Geometry check sheet. Reference: the model listing, model coordinates, mm. Face numbers are marked on the shaded views. A direction names the side the tool comes from. Give positions to 0.01 mm unless a question says otherwise; leave off trailing zeros. Order: outer loops, then holes, each group sorted by start corner. A loop starts at its lowest first (then second) coordinate and runs counter-clockwise, first axis right, second up.
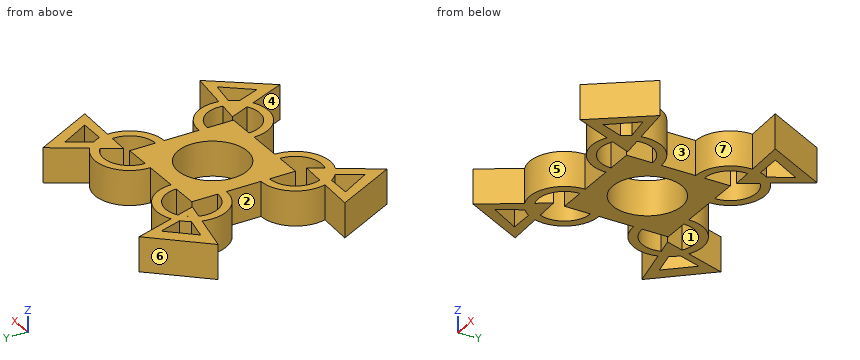
from build123d import *

# Parameters (mm, degrees)
F0_W     = 38.1
F0_H     = 38.1
F0_R     = 12.7
F1_DEPTH = 6.35
F2_R     = 12.7
F2_R_2   = 9.525
F3_DEPTH = 12.7
F5_DEPTH = 12.7


with BuildPart() as f1:
    # F0 (on Top) → F1 (new body, symmetric)
    with BuildSketch(Plane.XY):
        Rectangle(F0_W, F0_H)
        Circle(F0_R, mode=Mode.SUBTRACT)
    extrude(amount=F1_DEPTH, both=True)

    # F2 (on face) → F3 (join)
    with BuildSketch(Plane.XY.offset(6.35)):
        with Locations((-19.05, 19.05)):
            Circle(F2_R)
        with Locations((-19.05, 19.05)):
            Circle(F2_R_2, mode=Mode.SUBTRACT)
        with Locations((19.05, 19.05)):
            Circle(F2_R)
        with Locations((19.05, 19.05)):
            Circle(F2_R_2, mode=Mode.SUBTRACT)
        with Locations((19.05, -19.05)):
            Circle(F2_R)
        with Locations((19.05, -19.05)):
            Circle(F2_R_2, mode=Mode.SUBTRACT)
        with Locations((-19.05, -19.05)):
            Circle(F2_R)
        with Locations((-19.05, -19.05)):
            Circle(F2_R_2, mode=Mode.SUBTRACT)
    extrude(amount=-F3_DEPTH)

    # F4 (on face) → F5 (join)
    with BuildSketch(Plane.XY.offset(6.35)):
        Polygon((34.739992, 41.507824), (21.224035, 20.002501), (46.606169, 19.05), align=None)
        Polygon((40.44469, 22.77462), (27.74573, 22.937145), (34.235961, 33.853505), align=None, mode=Mode.SUBTRACT)
        Polygon((46.286524, -22.998363), (21.077219, -19.891765), (30.991478, -43.276963), align=None)
        Polygon((31.997671, -35.439923), (27.421833, -23.59291), (39.969566, -25.553625), align=None, mode=Mode.SUBTRACT)
        Polygon((-32.67766, -44.491031), (-19.05, -23.056319), (-44.426835, -21.971775), align=None)
        Polygon((-38.485192, -25.785192), (-25.785192, -25.785192), (-32.135192, -36.783715), align=None, mode=Mode.SUBTRACT)
        Polygon((-21.969239, 20.593261), (-29.732018, 44.777952), (-46.795185, 25.962843), align=None)
        Polygon((-30.201157, 36.994885), (-26.319768, 24.902539), (-38.732741, 27.58733), align=None, mode=Mode.SUBTRACT)
    extrude(amount=-F5_DEPTH)


solid = f1.part
Item 1: Set-up check for the marked faces 1, 2, 3 and 4: record each of +Z, -Z, +X, -X, +Y, -Y from which the full face is reachable in a straight line by a thin tool's end or side.
Reported:
face 1: +Z, -Z
face 2: +Z, -Z, -X
face 3: +Z, -Z, +X
face 4: +Z, -Z, -Y
Item 2: Scan lines: L1, parallel to Y at x = 0, z = 0.25; L2, parallel to X at y = -16, z = 1; L3, parallel to X at y = -17, z = 4.5. Record each from-to range of solid material in increasing order.
Reported:
L1: y = -19.05 to -12.7, 12.7 to 19.05
L2: x = -31.38 to -28.07, -19.05 to 19.05, 28.07 to 31.38
L3: x = -31.58 to -28.35, -19.05 to 19.05, 28.35 to 31.58
Item 3: Sectioned sample at C-C (x = 36). Enter the section's corners in (y, z), and give its area (3 significant figures).
Reported:
outline: (-36.64, -6.35) - (-30.48, -6.35) - (-30.48, 6.35) - (-36.64, 6.35) - close; (-24.93, -6.35) - (-21.73, -6.35) - (-21.73, 6.35) - (-24.93, 6.35) - close; (19.45, -6.35) - (22.83, -6.35) - (22.83, 6.35) - (19.45, 6.35) - close; (30.71, -6.35) - (39.12, -6.35) - (39.12, 6.35) - (30.71, 6.35) - close
area: 269 mm2
Item 4: Draft check along Y on the marked faces 5, 6 and 7. Enter one of: released by +Y, released by -Y, zero draft, split by the parting line, or undercut.
Reported:
face 5: released by -Y
face 6: released by +Y
face 7: undercut
Item 5: Sectioned sample at A-A (y = 0). Enter the section's corners in (x, z), and give its area (3 significant figures).
Reported:
outline: (-19.05, -6.35) - (-12.7, -6.35) - (-12.7, 6.35) - (-19.05, 6.35) - close; (12.7, -6.35) - (19.05, -6.35) - (19.05, 6.35) - (12.7, 6.35) - close
area: 161 mm2
Item 6: Sectioned sample at D-D (z = -1.5). Give the number of separate pieces and of enclosed holes in the cut face, and give its area (3 significant figures).
Reported:
separate pieces: 1
enclosed holes: 10
area: 2,350 mm2
Item 7: Gauge pin test, flat ends, axial feed: pin 1 (6.5 mm diameter, centred on x = 2.5, z = 0, fed in from +Y); pin 2 (3 mm diameter, centred on x = 15.5, z = -1, fed in from -Y); pin 3 (6 mm diameter, centred on y = -13, z = 2.5, fed in from -X); pin 4 (15 mm diameter, centred on x = 0, y = 0, fed in from -Z). Record the tip position at first contact, or that the pin passes through.
Reported:
pin 1: stops at y = 19.05
pin 2: stops at y = -31.58
pin 3: stops at x = -31.38
pin 4: passes through
